```python
from build123d import *

# Parameters (mm, degrees)
CYLINDER145_R             = 2.6
CYLINDER145_DEPTH         = 2
CYLINDER144_R             = 2.5
CYLINDER144_DEPTH         = 5
FUSION066_PLACEMENT_ANGLE = 90
CYLINDER153_R             = 2.6
CYLINDER153_DEPTH         = 2
CYLINDER152_R             = 2.5
CYLINDER152_DEPTH         = 5
FUSION070_PLACEMENT_ANGLE = 90
CYLINDER148_R             = 2.6
CYLINDER148_DEPTH         = 2
CYLINDER147_R             = 2.5
CYLINDER147_DEPTH         = 5
FUSION071_PLACEMENT_ANGLE = 90
CYLINDER139_R             = 2.6
CYLINDER139_DEPTH         = 2
CYLINDER138_R             = 2.5
CYLINDER138_DEPTH         = 5
FUSION064_PLACEMENT_ANGLE = 270
BOX037_W                  = 177
BOX037_H                  = 7
BOX037_DEPTH              = 18
BOX033_W                  = 7
BOX033_H                  = 22
BOX033_DEPTH              = 55
BOX034_W                  = 191
BOX034_H                  = 22
BOX034_DEPTH              = 7
BOX032_W                  = 7
BOX032_H                  = 22
BOX032_DEPTH              = 55


with BuildPart() as cilindro145:
    # Cylinder145 → Cylinder145 (new body)
    with BuildSketch(Plane.XY.offset(5)):
        Circle(CYLINDER145_R)
    extrude(amount=CYLINDER145_DEPTH)


with BuildPart() as obj1:
    # Cylinder144 → Cylinder144 (new body)
    with BuildSketch(Plane.XY):
        Circle(CYLINDER144_R)
    extrude(amount=CYLINDER144_DEPTH)

    # Fusion066: union Cilindro145
    add(cilindro145.part)


with BuildPart() as obj1_1:
    # Fusion066 placement: moved
    add(obj1.part.moved(Location((88.5, 29.5, 30))).rotate(Axis((88.5, 29.5, 30), (0, 1, 0)), FUSION066_PLACEMENT_ANGLE))


with BuildPart() as cilindro153:
    # Cylinder153 → Cylinder153 (new body)
    with BuildSketch(Plane.XY.offset(5)):
        Circle(CYLINDER153_R)
    extrude(amount=CYLINDER153_DEPTH)


with BuildPart() as obj2:
    # Cylinder152 → Cylinder152 (new body)
    with BuildSketch(Plane.XY):
        Circle(CYLINDER152_R)
    extrude(amount=CYLINDER152_DEPTH)

    # Fusion070: union Cilindro153
    add(cilindro153.part)


with BuildPart() as obj2_1:
    # Fusion070 placement: moved
    add(obj2.part.moved(Location((88.5, 44.5, 30))).rotate(Axis((88.5, 44.5, 30), (0, 1, 0)), FUSION070_PLACEMENT_ANGLE))


with BuildPart() as cilindro148:
    # Cylinder148 → Cylinder148 (new body)
    with BuildSketch(Plane.XY.offset(5)):
        Circle(CYLINDER148_R)
    extrude(amount=CYLINDER148_DEPTH)


with BuildPart() as obj3:
    # Cylinder147 → Cylinder147 (new body)
    with BuildSketch(Plane.XY):
        Circle(CYLINDER147_R)
    extrude(amount=CYLINDER147_DEPTH)

    # Fusion071: union Cilindro148
    add(cilindro148.part)


with BuildPart() as obj3_1:
    # Fusion071 placement: moved
    add(obj3.part.moved(Location((-88.5, 44.5, 30))).rotate(Axis((-88.5, 44.5, 30), (0, -1, 0)), FUSION071_PLACEMENT_ANGLE))


with BuildPart() as cilindro139:
    # Cylinder139 → Cylinder139 (new body)
    with BuildSketch(Plane.XY.offset(5)):
        Circle(CYLINDER139_R)
    extrude(amount=CYLINDER139_DEPTH)


with BuildPart() as fusion074:
    # Cylinder138 → Cylinder138 (new body)
    with BuildSketch(Plane.XY):
        Circle(CYLINDER138_R)
    extrude(amount=CYLINDER138_DEPTH)

    # Fusion064: union Cilindro139
    add(cilindro139.part)


with BuildPart() as fusion074_1:
    # Fusion064 placement: moved
    add(fusion074.part.moved(Location((-88.5, 29.5, 30))).rotate(Axis((-88.5, 29.5, 30), (0, 1, 0)), FUSION064_PLACEMENT_ANGLE))

    # Fusion074: union obj1, obj2, obj3
    add(obj1_1.part)
    add(obj2_1.part)
    add(obj3_1.part)


with BuildPart() as cubo034:
    # Box037 → Box037 (new body)
    with BuildSketch(Plane(origin=(-88.5, 26, 47), x_dir=(1, 0, 0), z_dir=(0, 0, 1))):
        with Locations((88.5, 3.5)):
            Rectangle(BOX037_W, BOX037_H)
    extrude(amount=BOX037_DEPTH)


with BuildPart() as cubo030:
    # Box033 → Box033 (new body)
    with BuildSketch(Plane(origin=(88.5, 26, 10), x_dir=(1, 0, 0), z_dir=(0, 0, 1))):
        with Locations((3.5, 11)):
            Rectangle(BOX033_W, BOX033_H)
    extrude(amount=BOX033_DEPTH)


with BuildPart() as cubo031:
    # Box034 → Box034 (new body)
    with BuildSketch(Plane(origin=(-95.5, 26, 65), x_dir=(1, 0, 0), z_dir=(0, 0, 1))):
        with Locations((95.5, 11)):
            Rectangle(BOX034_W, BOX034_H)
    extrude(amount=BOX034_DEPTH)


with BuildPart() as obj4:
    # Box032 → Box032 (new body)
    with BuildSketch(Plane(origin=(-95.5, 26, 10), x_dir=(1, 0, 0), z_dir=(0, 0, 1))):
        with Locations((3.5, 11)):
            Rectangle(BOX032_W, BOX032_H)
    extrude(amount=BOX032_DEPTH)

    # Fusion058: union Cubo034, Cubo030, Cubo031
    add(cubo034.part)
    add(cubo030.part)
    add(cubo031.part)

    # Cut058: cut Fusion074
    add(fusion074_1.part, mode=Mode.SUBTRACT)


solid = obj4.part
```
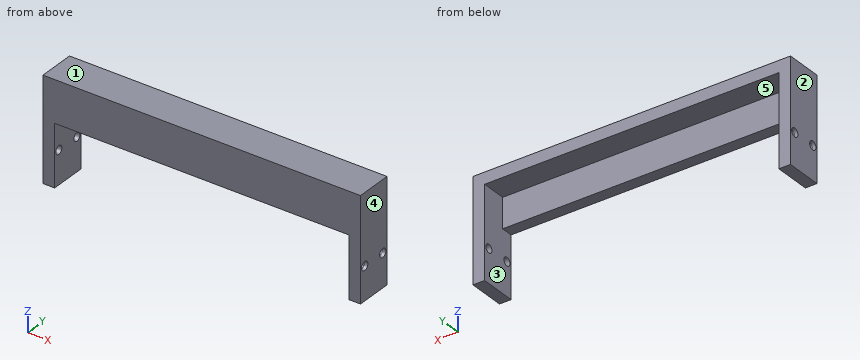
Here's how the part is built. I have some questions about the finished solid (model axes, mm). Face numbers are marked on the shaded views. A direction names the side the tool comes from. Round coordinates to 2 decimals unless told otherwise and drop trailing zeros. Loops run counter-clockwise (first coordinate to the right, second up) from the corner with the lowest first, then second, coordinate; pieces in that order, holes last. Notation, with made-up numbers: (74, 87.25) -> (112, 87.25) arc R12 cw to (112, 104.25) -> close; hole circle Ø11 at (87.5, -0.75). An arc over 180 degrees is marked (long way). Answer as CSV lines item,"result".
1. If we section it at D-D on y = 29.5: Please give me the cut outline in (x, z).
Final values:
outline,"(-95.5, 10) -> (-88.5, 10) -> (-88.5, 27.5) -> (-93.5, 27.5) -> (-93.5, 27.4) -> (-95.5, 27.4) -> close; (-95.5, 32.6) -> (-93.5, 32.6) -> (-93.5, 32.5) -> (-88.5, 32.5) -> (-88.5, 47) -> (88.5, 47) -> (88.5, 32.5) -> (93.5, 32.5) -> (93.5, 32.6) -> (95.5, 32.6) -> (95.5, 72) -> (-95.5, 72) -> close; (88.5, 10) -> (95.5, 10) -> (95.5, 27.4) -> (93.5, 27.4) -> (93.5, 27.5) -> (88.5, 27.5) -> close"
2. Which directions (+Z, -Z, +X, -X, +Y, -Y) give clear straight access to the entire face, cutting with the end or side of a thin tool? Please do the marked faces 4 and 5.
Final values:
face 4,"+Z, -Z, +X, +Y, -Y"
face 5,"-Z, +Y"
3. For pin 1 (14.5 mm diameter, centred on x = -8, z = 54.5, fed in from +Y); pin 2 (4.5 mm diameter, centred on x = -2.5, y = 38, fed in from -Z); pin 3 (3.5 mm diameter, centred on x = 6.5, y = 28, fed in from -Z); pin 4 (4.5 mm diameter, centred on y = 29.5, z = 30, fed in from -X), each with a flat end and sliding along its axis, tell me the tip position at first contact or that it passes through.
Final values:
pin 1,"stops at y = 33"
pin 2,"stops at z = 65"
pin 3,"stops at z = 47"
pin 4,"passes through"
4. If we section it at B-B on x = 62: Please give me the cut outline in (y, z), plus the area to 3 significant figures.
Final values:
outline,"(26, 47) -> (33, 47) -> (33, 65) -> (48, 65) -> (48, 72) -> (26, 72) -> close"
area,"280 mm^2"
5. If I drill on L1, parallel to Y at x = 94.1, z = 30; L2, parallel to Y at x = -90, z = 30; L3, parallel to X at y = 46.75, z = 56.5, over which ranges is the centre line in solid material (lowest first)?
Final values:
L1,"y = 26 to 26.9, 32.1 to 41.9, 47.1 to 48"
L2,"y = 26 to 27, 32 to 42, 47 to 48"
L3,"x = -95.5 to -88.5, 88.5 to 95.5"
6. If we section it at A-A on y = 44.5: Please give me the cut outline in (x, z).
Final values:
outline,"(-95.5, 10) -> (-88.5, 10) -> (-88.5, 27.5) -> (-93.5, 27.5) -> (-93.5, 27.4) -> (-95.5, 27.4) -> close; (-95.5, 32.6) -> (-93.5, 32.6) -> (-93.5, 32.5) -> (-88.5, 32.5) -> (-88.5, 65) -> (88.5, 65) -> (88.5, 32.5) -> (93.5, 32.5) -> (93.5, 32.6) -> (95.5, 32.6) -> (95.5, 72) -> (-95.5, 72) -> close; (88.5, 10) -> (95.5, 10) -> (95.5, 27.4) -> (93.5, 27.4) -> (93.5, 27.5) -> (88.5, 27.5) -> close"
7. Thinking about a two-plate mould opening in X: for the marked faces 1, 2 and 3, which applies, released by +X, released by -X, zero draft, split by the parting line, or undercut?
Final values:
face 1,"zero draft"
face 2,"released by -X"
face 3,"undercut"
8. If we section it at C-C on z = 49: Please give me the cut outline in (x, y), plus the area to 3 significant figures.
Final values:
outline,"(-95.5, 26) -> (95.5, 26) -> (95.5, 48) -> (88.5, 48) -> (88.5, 33) -> (-88.5, 33) -> (-88.5, 48) -> (-95.5, 48) -> close"
area,"1,550 mm^2"
